Design review of the part shown in the three views and the two pictorial views. Dimensions are in mm from the part's minimum x, y and z. A direction names the side the tool comes from. Give positions to 0.01 mm unless a question says otherwise; leave off trailing zeros. Loops run counter-clockwise (first coordinate to the right, second up) from the corner with the lowest first, then second, coordinate; pieces in that order, holes last. Notation, with made-up numbers: (-12.5, 10.5) - (-5.5, 10.5) arc R15 ccw to (-5.5, 15.5) - close; hole circle Ø3 at (71, 30.5). An arc over 180 degrees is marked (long way). Use CSV: the item, a comma, the result in double quotes. Start each with the question number.
1. For the marked faces 1 and 2, list the 3-axis set-ups (+Z, -Z, +X, -X, +Y, -Y) from which the entire face can be reached by the end or side of a thin tool; tool diameter is ignored.
2. Take a section at D-D on z = 14. Give the boundary of the cut face in (x, y), plus the area to 3 significant figures.
3. Take a section at C-C on x = 36. Give the boundary of the cut face in (y, z).
4. Take a section at A-A on y = 20. Give the boundary of the cut face in (x, z), plus the area to 3 significant figures.
5. Mouldability with a two-part tool opening along Z and no side actions: class the marked faces 3, 4 and 5 as pulls with the +Z half, pulls with the -Z half, needs draft (parallel to the pull), parting line crosses it, or undercut.
6. Take a section at B-B on z = 24. Give the boundary of the cut face in (x, y).
7. For pin 1 (8 mm diameter, centred on x = 36, y = 8.5, fed in from -Z); pin 2 (8 mm diameter, centred on x = 12.5, y = 12, fed in from +Z); pin 3 (21 mm diameter, centred on y = 20, z = 24, fed in from -X); pin 4 (6 mm diameter, centred on x = 28.5, y = 34.5, fed in from -Z), all flat-tipped, find the tip position at first contact; note any pin that passes through.
8. Wall thickness on line 1 (Z direction, x = 22, y = 20); line 2 (Y direction, x = 10, z = 24); line 3 (X direction, y = 6.5, z = 28.5): over which ranges is each line inside the solid? List them lowest first.
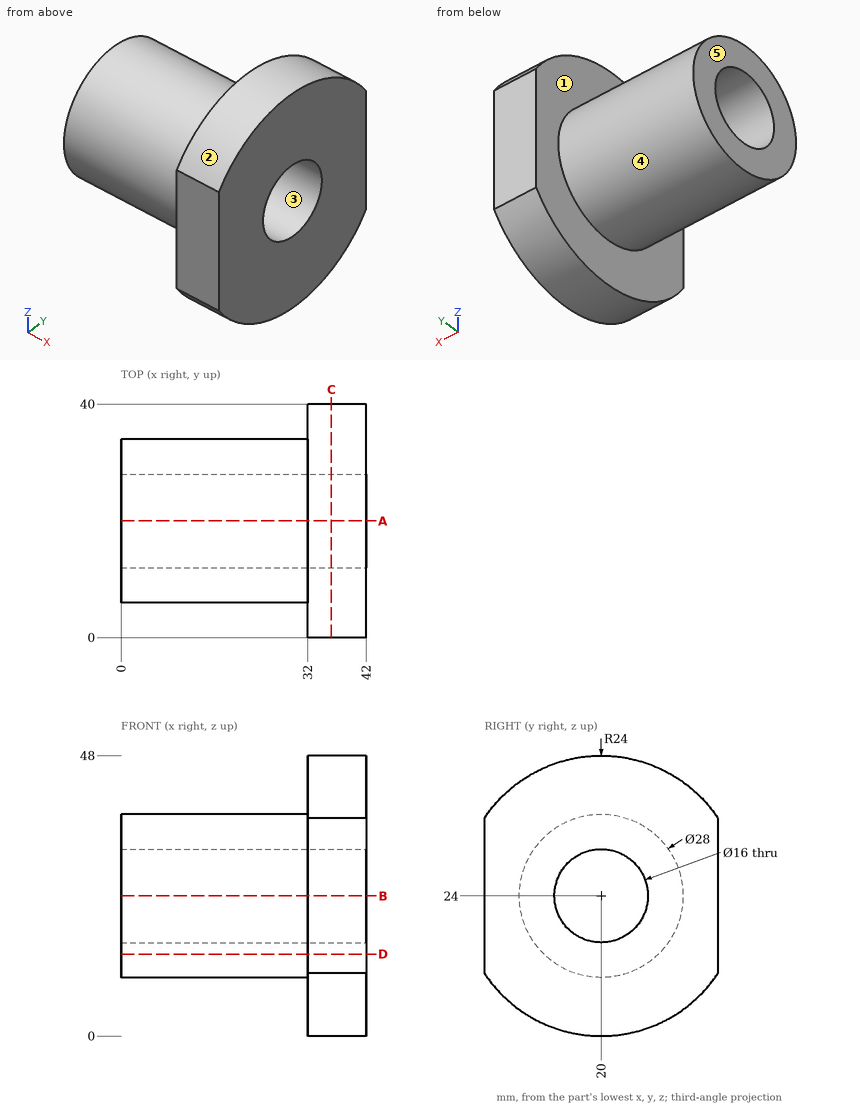
Check result:
1,face 1,"-X"
1,face 2,"+Z, +X, -X"
2,outline,"(0, 10.2) - (32, 10.2) - (32, 0) - (42, 0) - (42, 40) - (32, 40) - (32, 29.8) - (0, 29.8) - close"
2,area,"1,030 mm²"
3,outline,"(0, 10.73) arc R24 ccw to (40, 10.73) - (40, 37.27) arc R24 ccw to (0, 37.27) - close; hole circle Ø16 at (20, 24)"
4,outline,"(0, 10) - (32, 10) - (32, 0) - (42, 0) - (42, 16) - (0, 16) - close; (0, 32) - (42, 32) - (42, 48) - (32, 48) - (32, 38) - (0, 38) - close"
4,area,"704 mm²"
5,face 3,"undercut"
5,face 4,"parting line crosses it"
5,face 5,"needs draft"
6,outline,"(0, 6) - (32, 6) - (32, 0) - (42, 0) - (42, 12) - (0, 12) - close; (0, 28) - (42, 28) - (42, 40) - (32, 40) - (32, 34) - (0, 34) - close"
7,pin 1,"stops at z = 1.2"
7,pin 2,"stops at z = 37.42"
7,pin 3,"stops at x = 0"
7,pin 4,"stops at z = 16.02"
8,line 1,"z = 10 to 16, 32 to 38"
8,line 2,"y = 6 to 12, 28 to 34"
8,line 3,"x = 32 to 42"
